The model under review builds one solid part; all positions refer to its coordinate system, in mm. Face numbers are marked on the shaded views. A direction names the side the tool comes from. Round coordinates to 2 decimals unless told otherwise and drop trailing zeros. Loops run counter-clockwise (first coordinate to the right, second up) from the corner with the lowest first, then second, coordinate; pieces in that order, holes last. Notation, with made-up numbers: (12.25, 16) - (36.25, 16) arc R24 cw to (36.25, 29) - close; hole circle Ø6 at (65, 39.5). An arc over 180 degrees is marked (long way). Answer as CSV lines item,"result".
from build123d import *

# Parameters (mm, degrees)
SKETCH1_W                = 22.5
SKETCH1_H                = 19
BOSS_EXTRUDE1_DEPTH      = 63
FILLET1_R                = 2
BOSS_EXTRUDE2_DEPTH      = 10
BOSS_EXTRUDE2_DEPTH_BACK = 27.5
SKETCH2_R                = 2.75
SKETCH3_W                = 5
SKETCH3_H                = 3
BOSS_EXTRUDE3_DEPTH      = 6
SKETCH4_R                = 1.5
CUT_EXTRUDE1_DEPTH       = 10
SKETCH5_R                = 1.5
CUT_EXTRUDE2_DEPTH       = 73.912618935


with BuildPart() as part:
    # Sketch1 → Boss-Extrude1 (new body)
    with BuildSketch(Plane(origin=(0, 0, 0), x_dir=(1, 0, 0), z_dir=(0, 1, 0))):
        with Locations((11.25, 9.5)):
            Rectangle(SKETCH1_W, SKETCH1_H)
    extrude(amount=BOSS_EXTRUDE1_DEPTH)

    # Fillet1
    fillet1_edges = [part.edges().sort_by_distance(p)[0] for p in [
        (22.5, 0, -9.5),
        (0, 0, -9.5),
    ]]
    fillet(fillet1_edges, radius=FILLET1_R)

    # Sketch2 → Boss-Extrude2 (add, two sides: drawn at the far end of the back side and taken through both)
    with BuildSketch(Plane(origin=(0, 0, -19), x_dir=(-1, 0, 0), z_dir=(0, 0, -1)).offset(-BOSS_EXTRUDE2_DEPTH_BACK)):
        with Locations((-11.25, 11)):
            Circle(SKETCH2_R)
    extrude(amount=BOSS_EXTRUDE2_DEPTH + BOSS_EXTRUDE2_DEPTH_BACK)

    # Sketch3 → Boss-Extrude3 (add)
    with BuildSketch(Plane.XZ):
        with Locations((11.25, -8.517818065)):
            Rectangle(SKETCH3_W, SKETCH3_H)
    extrude(amount=BOSS_EXTRUDE3_DEPTH)

    # Sketch4 → Cut-Extrude1 (cut)
    with BuildSketch(Plane(origin=(0, 0, -10.017818065), x_dir=(-1, 0, 0), z_dir=(0, 0, -1))):
        with Locations((-11.25, -3)):
            Circle(SKETCH4_R)
    extrude(amount=-CUT_EXTRUDE1_DEPTH, mode=Mode.SUBTRACT)

    # Sketch5 → Cut-Extrude2 (cut, through all)
    with BuildSketch(Plane.XY):
        with Locations((20, 31)):
            Circle(SKETCH5_R)
        with Locations((2.5, 31)):
            Circle(SKETCH5_R)
    extrude(amount=-CUT_EXTRUDE2_DEPTH, mode=Mode.SUBTRACT)


solid = part.part
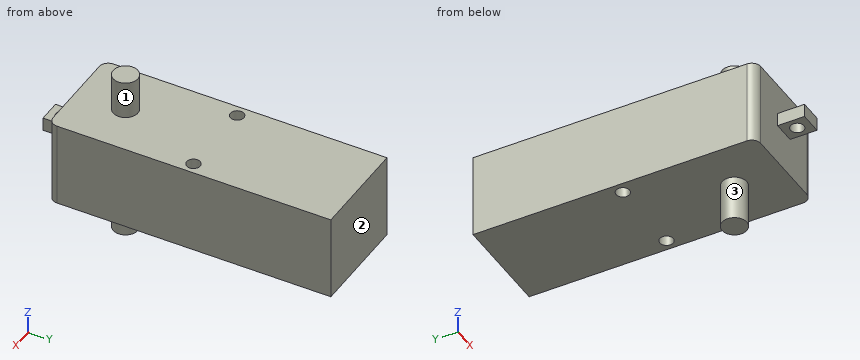
1. Take a section at A-A (y = 31). State the section outline as (x, z) points.
Numbers:
outline,"(0, -19) - (1, -19) - (1, 0) - (0, 0) - close; (4, -19) - (18.5, -19) - (18.5, 0) - (4, 0) - close; (21.5, -19) - (22.5, -19) - (22.5, 0) - (21.5, 0) - close"
2. Tool access review of the marked faces 1, 2 and 3: name each direction out of +Z, -Z, +X, -X, +Y, -Y from which nothing blocks a thin tool from reaching the whole face with its end or side.
Numbers:
face 1,"+Z"
face 2,"+Z, -Z, +X, -X, +Y"
face 3,"-Z"
3. Wall thickness on probe 1 along Z at (x, y) = (19.25, 18); probe 2 along Y at (x, z) = (17.25, -13); probe 3 along Y at (x, z) = (3, -1.5): over which ranges is each line inside the solid? List them lowest first.
Numbers:
probe 1,"z = -19 to 0"
probe 2,"y = 0 to 63"
probe 3,"y = 0 to 29.59, 32.41 to 63"
4. Take a section at D-D (y = -3). State the section outline as (x, z) points, plus the area to 3 significant figures.
Numbers:
outline,"(8.75, -10.02) - (9.75, -10.02) - (9.75, -7.02) - (8.75, -7.02) - close; (12.75, -10.02) - (13.75, -10.02) - (13.75, -7.02) - (12.75, -7.02) - close"
area,"6.00 mm²"
5. Clearance check with flat-ended pins moving along their axes: pin 1 (3 mm diameter, centred on x = 15.5, z = -15, fed in from -Y); pin 2 (1.5 mm diameter, centred on x = 14.5, y = 27, fed in from +Z); pin 3 (1.5 mm diameter, centred on y = -2.5, z = -8.5, fed in from +X); pin 4 (1.8 mm diameter, centred on x = 20, y = 31, fed in from +Z). State where each tip first meets the part, or that it passes through.
Numbers:
pin 1,"stops at y = 0"
pin 2,"stops at z = 0"
pin 3,"stops at x = 13.75"
pin 4,"passes through"
6. Take a section at C-C (z = -11). State the section outline as (x, y) points, plus the area to 3 significant figures.
Numbers:
outline,"(0, 2) arc R2 ccw to (2, 0) - (20.5, 0) arc R2 ccw to (22.5, 2) - (22.5, 63) - (0, 63) - close; hole circle Ø3 at (2.5, 31); hole circle Ø3 at (20, 31)"
area,"1,400 mm²"
7. Take a section at B-B (x = 11.25). State the section outline as (y, z) points.
Numbers:
outline,"(-6, -10.02) - (-4.5, -10.02) - (-4.5, -7.02) - (-6, -7.02) - close; (-1.5, -10.02) - (0, -10.02) - (0, -19) - (8.25, -19) - (8.25, -29) - (13.75, -29) - (13.75, -19) - (63, -19) - (63, 0) - (13.75, 0) - (13.75, 8.5) - (8.25, 8.5) - (8.25, 0) - (0, 0) - (0, -7.02) - (-1.5, -7.02) - close"
